Geometry: see drawing. Coordinates: mm, zero at the bounding-box minimum. Give positions to 0.01 mm unless a question says otherwise; leave off trailing zeros. Write each loop counter-clockwise with the first axis right and the second up, starting at its lowest first coordinate (ties: lowest second). Pieces come first, ordered by that corner, then holes. Notation, with made-up numbers: (36, 50.5) - (45, 50.5) arc R5 cw to (45, 55.5) - close; hole circle Ø2 at (29, 37.25). An arc over 180 degrees is marked (long way). Use CSV: the item, a comma, the result in double quotes. Start each with the question number.
(1) First-contact query: pin 1 Ø1.5 at (x, y) = (84.5, 2.5) entering from -Z; pin 2 Ø2.5 at (y, z) = (1.5, 26) entering from +X; pin 3 Ø1.5 at (y, z) = (3.5, 18) entering from -X. Flat tips, straight axial feed; report the tip coordinate or a pass-through.
(2) Section C-C on y = 4.2. Output: boundary loops of the cut face in (x, z) (1 decimal), and give its area (3 significant figures).
(3) Line query: probe 1 along X at (y, z) = (3.2, 24.5); probe 2 along Z at (x, y) = (27, 1.4); probe 3 along Z at (x, y) = (91.5, 1.2). Output: solid intervals per line, ascending. Write a range as [from, to].
(4) Section B-B on z = 32.5. Output: boundary loops of the cut face in (x, y).
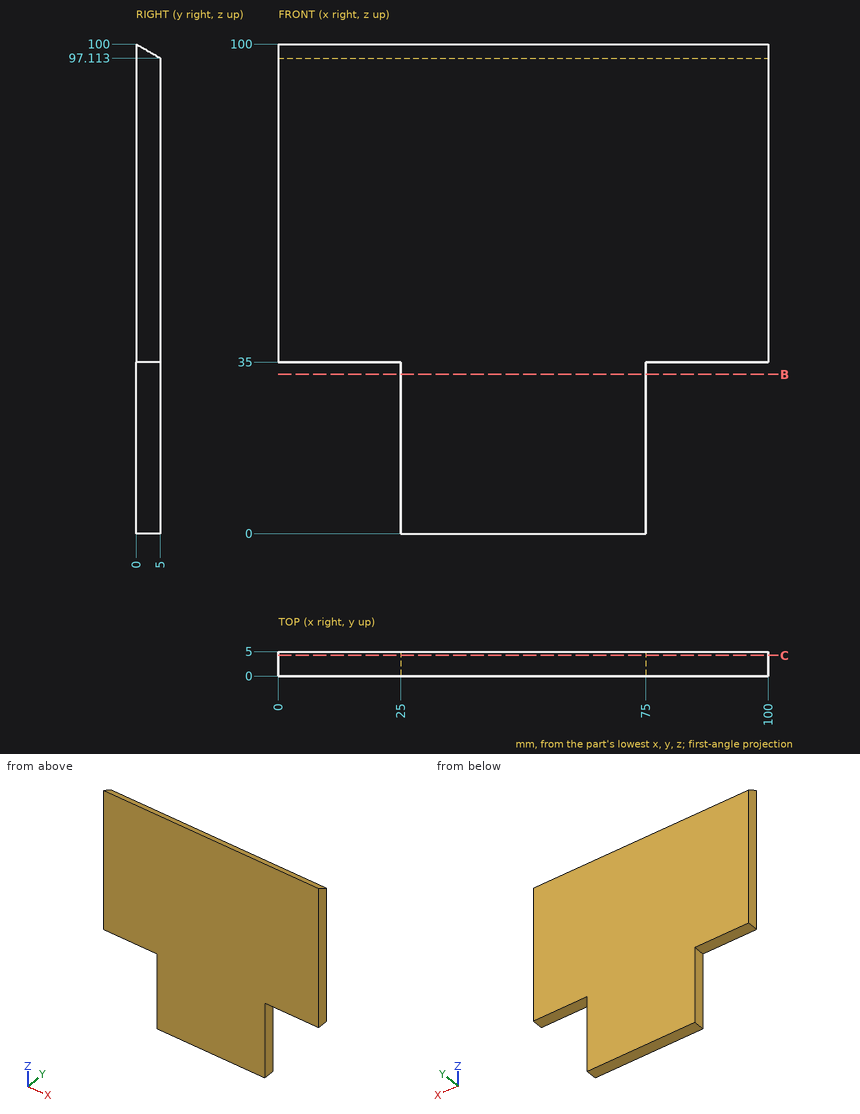
Check values:
1,pin 1,"stops at z = 35"
1,pin 2,"stops at x = 75"
1,pin 3,"stops at x = 25"
2,outline,"(0, 35) - (25, 35) - (25, 0) - (75, 0) - (75, 35) - (100, 35) - (100, 97.6) - (0, 97.6) - close"
2,area,"8,010 mm²"
3,probe 1,"x = [25, 75]"
3,probe 2,"z = [0, 99.19]"
3,probe 3,"z = [35, 99.31]"
4,outline,"(25, 0) - (75, 0) - (75, 5) - (25, 5) - close"
